Autodesk Inventor part; units mm, degrees
ref_plane "YZ Plane" through (0, 0, 0) normal (1, 0, 0) x (0, 1, 0)
ref_plane "XZ Plane" through (0, 0, 0) normal (0, 1, 0) x (-1, 0, 0)
ref_plane "XY Plane" through (0, 0, 0) normal (0, 0, 1) x (1, 0, 0)
sketch "Sketch1" plane through (0, 0, 0) normal (0, 1, 0) x (-1, 0, 0)
  line L0 (0, -5.4) -> (1.5, -5.4)
  line L1 (1.5, -5.4) -> (1.5, -8.1)
  line L2 (1.5, -8.1) -> (3.2, -8.1)
  line L3 (0, 0) -> (1.5, 0)
  line L4 (1.5, 0) -> (1.5, 2.7)
  line L5 (1.5, 2.7) -> (3.2, 2.7)
  line L6 (5, 0) -> (5, -5.4)
  line L7 (5, -5.4) -> (3.2, -8.1)
  line L8 (5, 0) -> (3.2, 2.7)
  line L9 (0, -20) -> (1.5, -20)
  line L10 (1.5, -20) -> (1.5, -17.3)
  line L11 (1.5, -17.3) -> (3.2, -17.3)
  line L12 (0, -25.4) -> (1.5, -25.4)
  line L13 (1.5, -25.4) -> (1.5, -28.1)
  line L14 (1.5, -28.1) -> (3.2, -28.1)
  line L15 (5, -20) -> (5, -25.4)
  line L16 (5, -25.4) -> (3.2, -28.1)
  line L17 (5, -20) -> (3.2, -17.3)
  line L18 (0, -5.4) -> (0, -20)
  line L19 (0, 0) -> (0, 7.3)
  line L20 (0, 7.3) -> (-5, 7.3)
  line L21 (0, -25.4) -> (0, -32.7)
  line L22 (0, -32.7) -> (-5, -32.7)
  line L23 (-5, -32.7) -> (-5, 7.3)
  dimension "d0" = 5.4
  dimension "d1" = 1.5
  dimension "d2" = 2.7
  dimension "d3" = 1.7
  dimension "d4" = 2.7
  dimension "d5" = 1.7
  dimension "d9" = 2.7
  dimension "d10" = 2.7
  dimension "d11" = 5.4
  dimension "d12" = 7.3
  dimension "d13" = 5
  dimension "d14" = 7.3
  dimension "d15" = 5
  dimension "d16" = 20
extrude "Extrusion1" add sketch "Sketch1" along normal blind 40
sketch "Sketch2" plane through (5, 0, 7.3) normal (1, 0, 0) x (0, 0, -1)
  line L0 (11.6599, 5) -> (8.3401, 5)
  line L1 (8.3401, 5) -> (6.6802, 7.875)
  line L2 (6.6802, 7.875) -> (8.3401, 10.75)
  line L3 (8.3401, 10.75) -> (11.6599, 10.75)
  line L4 (11.6599, 10.75) -> (13.3198, 7.875)
  line L5 (13.3198, 7.875) -> (11.6599, 5)
  line L6 (40, 0) -> (0, 0)
  line L7 (0, 0) -> (0, 40)
  line L8 (31.6599, 5) -> (28.3401, 5)
  line L9 (28.3401, 5) -> (26.6802, 7.875)
  line L10 (26.6802, 7.875) -> (28.3401, 10.75)
  line L11 (28.3401, 10.75) -> (31.6599, 10.75)
  line L12 (31.6599, 10.75) -> (33.3198, 7.875)
  line L13 (33.3198, 7.875) -> (31.6599, 5)
  line L14 (40, 0) -> (40, 40)
  line L15 (11.6599, 29.25) -> (8.3401, 29.25)
  line L16 (8.3401, 29.25) -> (6.6802, 32.125)
  line L17 (6.6802, 32.125) -> (8.3401, 35)
  line L18 (8.3401, 35) -> (11.6599, 35)
  line L19 (11.6599, 35) -> (13.3198, 32.125)
  line L20 (13.3198, 32.125) -> (11.6599, 29.25)
  line L21 (31.6599, 29.25) -> (28.3401, 29.25)
  line L22 (28.3401, 29.25) -> (26.6802, 32.125)
  line L23 (26.6802, 32.125) -> (28.3401, 35)
  line L24 (28.3401, 35) -> (31.6599, 35)
  line L25 (31.6599, 35) -> (33.3198, 32.125)
  line L26 (33.3198, 32.125) -> (31.6599, 29.25)
  line L27 (0, 40) -> (40, 40)
  point P0 (7.3, 0)
  point P1 (10, 7.875)
  point P2 (30, 7.875)
  point P3 (10, 32.125)
  point P4 (30, 32.125)
  dimension "d17" = 5.75
  dimension "d18" = 5
  dimension "d19" = 10
  dimension "d20" = 5.75
  dimension "d21" = 5
  dimension "d22" = 10
  dimension "d23" = 5.75
  dimension "d24" = 5.75
  dimension "d25" = 5
  dimension "d26" = 5
  dimension "d27" = 10
  dimension "d28" = 10
extrude "Extrusion2" cut sketch "Sketch2" against normal blind 2.5 contours L0 L1 L2 L3 L4 L5 | L8 L9 L10 L11 L12 L13 | L15 L16 L17 L18 L19 L20 | L21 L22 L23 L24 L25 L26
sketch "Sketch3" plane through (2.5, 0, 7.3) normal (1, 0, 0) x (0, 0, -1)
  circle A0 centre (30, 7.75) radius 1.375
  circle A1 centre (10, 7.75) radius 1.375
  circle A2 centre (10, 32.25) radius 1.375
  circle A3 centre (30, 32.25) radius 1.375
  point P0 (7.3, 0)
  dimension "d31" = 2.75
  dimension "d32" = 2.75
  dimension "d33" = 2.75
extrude "Extrusion3" cut sketch "Sketch3" against normal blind 20
properties part number "slotmountingPlate_dual_m3"
Design review of the part built by this model. Coordinates are the model's own, in mm. A direction names the side the tool comes from. Coordinates: 2 decimals unless noted, no trailing zeros. Loops run counter-clockwise (first coordinate to the right, second up) from the corner with the lowest first, then second, coordinate; pieces in that order, holes last. Notation, with made-up numbers: (78.25, 76.5) -> (121.25, 76.5) arc R14 ccw to (121.25, 88.5) -> close; hole circle Ø8 at (39, 23.25). An arc over 180 degrees is marked (long way). Answer as a JSON object with one key per item and string values.
Q1. The part is to be moulded in two halves that separate along Y. For faces 6 (the flat face through (-1, 20, -5.4)), 7 (the flat face through (3.768, 9.292, -20.199)), say which applies: +Y half, -Y half, draft (parallel to the pull), parting line (faces both ways), or undercut.
Answer block:
{"face 6": "draft", "face 7": "undercut"}
Q2. Take a section at C-C on x = 3.25. Give the boundary of the cut face in (y, z) (3 decimals), plus the area to 3 significant figures.
Answer block:
{"outline": "(0, -32.7) -> (40, -32.7) -> (40, 7.3) -> (0, 7.3) -> close; hole (5, -24.36) -> (7.875, -26.02) -> (10.75, -24.36) -> (10.75, -21.04) -> (7.875, -19.38) -> (5, -21.04) -> close; hole (5, -4.36) -> (7.875, -6.02) -> (10.75, -4.36) -> (10.75, -1.04) -> (7.875, 0.62) -> (5, -1.04) -> close; hole (29.25, -24.36) -> (32.125, -26.02) -> (35, -24.36) -> (35, -21.04) -> (32.125, -19.38) -> (29.25, -21.04) -> close; hole (29.25, -4.36) -> (32.125, -6.02) -> (35, -4.36) -> (35, -1.04) -> (32.125, 0.62) -> (29.25, -1.04) -> close", "area": "1,490 mm^2"}
Q3. Take a section at B-B on z = -2.7. Give the boundary of the cut face in (x, y) (3 decimals), plus the area to 3 significant figures.
Answer block:
{"outline": "(-5, 0) -> (5, 0) -> (5, 5) -> (2.5, 5) -> (2.5, 6.375) -> (-5, 6.375) -> close; (-5, 9.125) -> (2.5, 9.125) -> (2.5, 10.75) -> (5, 10.75) -> (5, 29.25) -> (2.5, 29.25) -> (2.5, 30.875) -> (-5, 30.875) -> close; (-5, 33.625) -> (2.5, 33.625) -> (2.5, 35) -> (5, 35) -> (5, 40) -> (-5, 40) -> close", "area": "330 mm^2"}
Q4. Tool access review of faces 1 (the flat face through (-1, 20, 0)), 2 (the flat face through (3.77, 33.58, -5.18)), 3 (the flat face through (0, 20, -13)), 4 (the flat face through (-4.113, 19.72, -26.731)), 5 (the cylindrical face through (-1.197, 33.613, -22.521)): name each direction out of +Z, -Z, +X, -X, +Y, -Y from which nothing blocks a thin tool from reaching the whole face with its end or side.
Answer block:
{"face 1": "+Z, +Y, -Y", "face 2": "+X", "face 3": "+Y, -Y", "face 4": "-Z, -X, +Y, -Y", "face 5": "+X, -X"}
Q5. Take a section at D-D on z = -7. Give the boundary of the cut face in (x, y).
Answer block:
{"outline": "(-3.93, 0) -> (-1.5, 0) -> (-1.5, 40) -> (-3.93, 40) -> close; (0, 0) -> (5, 0) -> (5, 40) -> (0, 40) -> close"}
Q6. Clearance check with flat-ended pins moving along their axes: pin 1 Ø1.4 at (x, y) = (-2.5, 28.5) entering from -Z; pin 2 Ø0.8 at (x, y) = (-0.5, 16.5) entering from -Z; pin 3 Ø4.5 at (y, z) = (20.5, -15.5) entering from -X. State where each tip first meets the part, or that it passes through.
Answer block:
{"pin 1": "stops at z = -28.1", "pin 2": "stops at z = -25.4", "pin 3": "stops at x = -3.5"}
Q7. Take a section at A-A on x = -4. Give the boundary of the cut face in (y, z) (3 decimals), plus the area to 3 significant figures.
Answer block:
{"outline": "(0, -26.9) -> (40, -26.9) -> (40, -18.5) -> (0, -18.5) -> close; (0, -6.9) -> (40, -6.9) -> (40, 1.5) -> (0, 1.5) -> close; hole circle Ø2.75 at (7.75, -22.7); hole circle Ø2.75 at (7.75, -2.7); hole circle Ø2.75 at (32.25, -22.7); hole circle Ø2.75 at (32.25, -2.7)", "area": "648 mm^2"}
Q8. To check wall thickness, follow L1, parallel to Y at x = -2.5, z = -2.7 (3 decimals); L2, parallel to Z at x = -2.5, y = 35; L3, parallel to Z at x = 4.5, y = 9. State the ranges of each line that lie inside material, in increasing order.
Answer block:
{"L1": "y = 0 to 6.375, 9.125 to 30.875, 33.625 to 40", "L2": "z = -28.1 to -17.3, -8.1 to 2.7", "L3": "z = -32.7 to -25.37, -20.03 to -5.37, -0.03 to 7.3"}
